```python
from build123d import *

# Parameters (mm, degrees)
BOSS_EXTRUDE1_DEPTH = 19.25
SKETCH2_R           = 2.875
BOSS_EXTRUDE2_DEPTH = 4
CUT_EXTRUDE1_REACH  = 60.727
SKETCH3_R           = 2


with BuildPart() as part:
    # Sketch1 → Boss-Extrude1 (new body)
    with BuildSketch(Plane.XY):
        Polygon((0, 0), (40.8, 0), (40.8, 26.8), (46.8, 26.8), (46.8, 29.8), (40.8, 29.8), (40.8, 39), (0, 39), (0, 29.8), (-6, 29.8), (-6, 26.8), (0, 26.8), align=None)
    extrude(amount=BOSS_EXTRUDE1_DEPTH)

    # Sketch2 → Boss-Extrude2 (add)
    with BuildSketch(Plane(origin=(0, 39, 0), x_dir=(1, 0, 0), z_dir=(0, 1, 0))):
        with Locations((31.175, -9.625)):
            Circle(SKETCH2_R)
    extrude(amount=BOSS_EXTRUDE2_DEPTH)

    # Sketch3 → Cut-Extrude1 (cut, up to next)
    with BuildSketch(Plane(origin=(0, 29.8, 0), x_dir=(1, 0, 0), z_dir=(0, 1, 0)), mode=Mode.PRIVATE) as cut_extrude1_sk1:
        with Locations((45.15, -15)):
            Circle(SKETCH3_R)
    cut_extrude1_tool1 = extrude(cut_extrude1_sk1.sketch, amount=-CUT_EXTRUDE1_REACH, mode=Mode.PRIVATE) & part.part
    # Sketch3 → Cut-Extrude1 (cut, up to next)
    with BuildSketch(Plane(origin=(0, 29.8, 0), x_dir=(1, 0, 0), z_dir=(0, 1, 0)), mode=Mode.PRIVATE) as cut_extrude1_sk2:
        with Locations((45.15, -4.25)):
            Circle(SKETCH3_R)
    cut_extrude1_tool2 = extrude(cut_extrude1_sk2.sketch, amount=-CUT_EXTRUDE1_REACH, mode=Mode.PRIVATE) & part.part
    # Sketch3 → Cut-Extrude1 (cut, up to next)
    with BuildSketch(Plane(origin=(0, 29.8, 0), x_dir=(1, 0, 0), z_dir=(0, 1, 0)), mode=Mode.PRIVATE) as cut_extrude1_sk3:
        with Locations((-4.35, -4.25)):
            Circle(SKETCH3_R)
    cut_extrude1_tool3 = extrude(cut_extrude1_sk3.sketch, amount=-CUT_EXTRUDE1_REACH, mode=Mode.PRIVATE) & part.part
    # Sketch3 → Cut-Extrude1 (cut, up to next)
    with BuildSketch(Plane(origin=(0, 29.8, 0), x_dir=(1, 0, 0), z_dir=(0, 1, 0)), mode=Mode.PRIVATE) as cut_extrude1_sk4:
        with Locations((-4.35, -15)):
            Circle(SKETCH3_R)
    cut_extrude1_tool4 = extrude(cut_extrude1_sk4.sketch, amount=-CUT_EXTRUDE1_REACH, mode=Mode.PRIVATE) & part.part
    add(cut_extrude1_tool1.solids().sort_by_distance((45.15, 29.8, 15))[0], mode=Mode.SUBTRACT)
    add(cut_extrude1_tool2.solids().sort_by_distance((45.15, 29.8, 4.25))[0], mode=Mode.SUBTRACT)
    add(cut_extrude1_tool3.solids().sort_by_distance((-4.35, 29.8, 4.25))[0], mode=Mode.SUBTRACT)
    add(cut_extrude1_tool4.solids().sort_by_distance((-4.35, 29.8, 15))[0], mode=Mode.SUBTRACT)


solid = part.part
```
Work out the finished part from the listing and answer in its coordinate system (mm). A direction names the side the tool comes from. Give positions to 0.01 mm unless a question says otherwise; leave off trailing zeros. Write each loop counter-clockwise with the first axis right and the second up, starting at its lowest first coordinate (ties: lowest second). Pieces come first, ordered by that corner, then holes. Notation, with made-up numbers: (31.5, 32.25) - (73.5, 32.25) arc R26 ccw to (73.5, 57.25) - close; hole circle Ø2 at (-38, -0.75). An arc over 180 degrees is marked (long way). Use one line per item in the form item = value.
1. A cutting plane is placed at C-C (y = 6). Write down the section's boundary in (x, z), and give its area (3 significant figures).
Filled in:
outline = (0, 0) - (40.8, 0) - (40.8, 19.25) - (0, 19.25) - close
area = 785 mm^2
2. For faces 1 (the face through (0, 14, 9)), 2 (the face through (40.8, 34, 9)), 3 (the face through (0, 34, 9)), determine the directions among +Z, -Z, +X, -X, +Y, -Y from which every point of the face is accessible in a straight line to the end or side of a thin tool.
Filled in:
face_1 = +Z, -Z, -X, -Y
face_2 = +Z, -Z, +X, +Y
face_3 = +Z, -Z, -X, +Y
3. A cutting plane is placed at A-A (x = 45.15). Write down the section's boundary in (y, z).
Filled in:
outline = (26.8, 0) - (29.8, 0) - (29.8, 2.25) - (26.8, 2.25) - close; (26.8, 6.25) - (29.8, 6.25) - (29.8, 13) - (26.8, 13) - close; (26.8, 17) - (29.8, 17) - (29.8, 19.25) - (26.8, 19.25) - close
4. A cutting plane is placed at B-B (z = 15). Write down the section's boundary in (x, y), and give its area (3 significant figures).
Filled in:
outline = (-2.35, 26.8) - (0, 26.8) - (0, 0) - (40.8, 0) - (40.8, 26.8) - (43.15, 26.8) - (43.15, 29.8) - (40.8, 29.8) - (40.8, 39) - (0, 39) - (0, 29.8) - (-2.35, 29.8) - close
area = 1,610 mm^2
5. Consider L1, parallel to Z at x = -4.35, y = 28.25; L2, parallel to X at y = 13, z = 11.25; L3, parallel to Y at x = 18.5, z = 8.75. Determine where each line is inside the solid, lowest interval first.
Filled in:
L1 = 0 to 2.25, 6.25 to 13, 17 to 19.25
L2 = 0 to 40.8
L3 = 0 to 39
6. Determine the mould class of faces 4 (the face through (43, 26.8, 9)), 5 (the face through (33.83, 40.97, 10.73)), 6 (the face through (-2.35, 28.32, 4.32)), 7 (the face through (-6, 28, 10)) for opening direction X: released by +X, released by -X, zero draft, split by the parting line, or undercut.
Filled in:
face_4 = zero draft
face_5 = split by the parting line
face_6 = undercut
face_7 = released by -X
7. Each of these flat-tipped pins is pushed along its axis until it touches: pin 1 Ø6.5 at (x, z) = (45.15, 4.25) entering from +Y; pin 2 Ø3 at (x, z) = (45.15, 15) entering from +Y; pin 3 Ø1.8 at (x, z) = (43, 13) entering from -Y; pin 4 Ø5 at (y, z) = (13.5, 13.5) entering from -X. Where does it stop, or does it pass through?
Filled in:
pin_1 = 29.8
pin_2 = through
pin_3 = 26.8
pin_4 = 0
8. A cutting plane is placed at D-D (x = 37). Write down the section's boundary in (y, z).
Filled in:
outline = (0, 0) - (39, 0) - (39, 19.25) - (0, 19.25) - close
